```python
from build123d import *
from OCP.BRepFilletAPI import BRepFilletAPI_MakeFillet

# Parameters (mm, degrees)
SKETCH1_R                = 1.5
BOSS_EXTRUDE1_DEPTH      = 1.5
BOSS_EXTRUDE2_DEPTH      = 2
BOSS_EXTRUDE2_DEPTH_BACK = 1.5
SKETCH3_W                = 5
SKETCH3_H                = 0.7
SKETCH4_W                = 5
SKETCH4_H                = 1.5
BOSS_EXTRUDE3_DEPTH      = 0.15
FILLET2_R                = 0.85
SKETCH5_W                = 5
SKETCH5_H                = 1.2
BOSS_EXTRUDE4_DEPTH      = 2.5
BOSS_EXTRUDE4_2_DEPTH    = 2.5
SKETCH6_W                = 4
SKETCH6_H                = 5
BOSS_EXTRUDE5_DEPTH      = 2.35
FILLET3_R                = 1.5
CUT_EXTRUDE1_DEPTH       = 2.5
FILLET4_R1               = 3
FILLET4_R2               = 1


with BuildPart() as part:
    # Sketch1 → Boss-Extrude1 (new body)
    with BuildSketch(Plane(origin=(0, 0, 0), x_dir=(1, 0, 0), z_dir=(0, 1, 0))):
        with BuildLine():
            Line((0, 0), (43, 0))
            Line((43, 0), (43, 36))
            Line((43, 36), (43, 41))
            ThreePointArc((43, 41), (39, 45), (35, 41))
            Line((35, 41), (35, 36))
            Line((35, 36), (0, 36))
            Line((0, 36), (0, 0))
        make_face()
        with Locations(Location((39, 41, 0), (0, 0, 270))):
            Circle(SKETCH1_R, mode=Mode.SUBTRACT)
    extrude(amount=BOSS_EXTRUDE1_DEPTH)



with BuildPart() as body_2:
    # Sketch3 → Boss-Extrude2 (new, two sides: drawn at the far end of the back side and taken through both)
    with BuildSketch(Plane.XY.offset(-BOSS_EXTRUDE2_DEPTH_BACK)):
        with Locations((39, 2)):
            Rectangle(SKETCH3_W, SKETCH3_H)
    extrude(amount=BOSS_EXTRUDE2_DEPTH + BOSS_EXTRUDE2_DEPTH_BACK)


with BuildPart() as part_1:
    add(part.part)

    add(body_2.part)  # Boss-Extrude3 merges body 2
    # Sketch4 → Boss-Extrude3 (add)
    with BuildSketch(Plane.XZ.offset(-1.65)):
        with Locations((39, -0.75)):
            Rectangle(SKETCH4_W, SKETCH4_H)
    extrude(amount=BOSS_EXTRUDE3_DEPTH)

    # Fillet2
    fillet2_edges = [part_1.edges().sort_by_distance(p)[0] for p in [
        (39, 1.5, -1.5),
    ]]
    fillet(fillet2_edges, radius=FILLET2_R - 0.0001)  # a hair under: the kernel refuses the full size



with BuildPart() as body_2_2:
    # Sketch5 → Boss-Extrude4 (new body)
    with BuildSketch(Plane.ZY):
        with Locations((-10, 3.25)):
            Rectangle(SKETCH5_W, SKETCH5_H)
    extrude(amount=BOSS_EXTRUDE4_DEPTH)


with BuildPart() as body_3:
    # Sketch5 → Boss-Extrude4 2 (new body)
    with BuildSketch(Plane.ZY):
        with Locations((-26, 3.25)):
            Rectangle(SKETCH5_W, SKETCH5_H)
    extrude(amount=BOSS_EXTRUDE4_2_DEPTH)


with BuildPart() as part_2:
    add(part_1.part)

    add(body_2_2.part)  # Boss-Extrude5 merges body 2 2

    add(body_3.part)  # Boss-Extrude5 merges body 3
    # Sketch6 → Boss-Extrude5 (add)
    with BuildSketch(Plane(origin=(0, 1.5, 0), x_dir=(1, 0, 0), z_dir=(0, 1, 0))):
        with Locations((2, 26)):
            Rectangle(SKETCH6_W, SKETCH6_H)
        with Locations((2, 10)):
            Rectangle(SKETCH6_W, SKETCH6_H)
    extrude(amount=BOSS_EXTRUDE5_DEPTH)

    # Fillet3
    fillet3_edges = [part_2.edges().sort_by_distance(p)[0] for p in [
        (2, 1.5, -7.5),
    ]]
    fillet(fillet3_edges, radius=FILLET3_R)
    fillet3_2_edges = [part_2.edges().sort_by_distance(p)[0] for p in [
        (4, 1.5, -10),
    ]]
    fillet(fillet3_2_edges, radius=FILLET3_R)
    fillet3_3_edges = [part_2.edges().sort_by_distance(p)[0] for p in [
        (2, 1.5, -12.5),
    ]]
    fillet(fillet3_3_edges, radius=FILLET3_R)
    fillet3_4_edges = [part_2.edges().sort_by_distance(p)[0] for p in [
        (2, 1.5, -23.5),
    ]]
    fillet(fillet3_4_edges, radius=FILLET3_R)
    fillet3_5_edges = [part_2.edges().sort_by_distance(p)[0] for p in [
        (4, 1.5, -26),
    ]]
    fillet(fillet3_5_edges, radius=FILLET3_R - 0.0001)  # a hair under: the kernel refuses the full size
    fillet3_6_edges = [part_2.edges().sort_by_distance(p)[0] for p in [
        (2, 1.5, -28.5),
    ]]
    fillet(fillet3_6_edges, radius=FILLET3_R - 0.0001)  # a hair under: the kernel refuses the full size

    # Sketch7 → Cut-Extrude1 (cut)
    with BuildSketch(Plane(origin=(0, 1.5, 0), x_dir=(1, 0, 0), z_dir=(0, 1, 0))):
        Polygon((13.196152423, 29), (8, 32), (8, 26), align=None)
        Polygon((17, 26), (22.196152423, 29), (17, 32), align=None)
        Polygon((26, 26), (31.196152423, 29), (26, 32), align=None)
        Polygon((35, 26), (40.196152423, 29), (35, 32), align=None)
        Polygon((13.196152423, 18), (8, 21), (8, 15), align=None)
        Polygon((17, 15), (22.196152423, 18), (17, 21), align=None)
        Polygon((26, 15), (31.196152423, 18), (26, 21), align=None)
        Polygon((35, 15), (40.196152423, 18), (35, 21), align=None)
        Polygon((13.196152423, 7), (8, 10), (8, 4), align=None)
        Polygon((17, 4), (22.196152423, 7), (17, 10), align=None)
        Polygon((26, 4), (31.196152423, 7), (26, 10), align=None)
        Polygon((35, 4), (40.196152423, 7), (35, 10), align=None)
        Polygon((9.5, 23.5), (14.696152423, 26.5), (14.696152423, 20.5), align=None)
        Polygon((23.696152423, 20.5), (18.5, 23.5), (23.696152423, 26.5), align=None)
        Polygon((32.696152423, 20.5), (27.5, 23.5), (32.696152423, 26.5), align=None)
        Polygon((14.696152423, 9.5), (9.5, 12.5), (14.696152423, 15.5), align=None)
        Polygon((18.5, 12.5), (23.696152423, 15.5), (23.696152423, 9.5), align=None)
        Polygon((32.696152423, 9.5), (27.5, 12.5), (32.696152423, 15.5), align=None)
    extrude(amount=-CUT_EXTRUDE1_DEPTH, mode=Mode.SUBTRACT)

    # Fillet4: one fillet with a radius per group of edges: ONE call of the kernel's fillet builder (fillet() takes one radius for all edges)
    fillet4_edges_1 = [part_2.edges().sort_by_distance(p)[0] for p in [
        (0, 0.75, 0),
        (0, 0.75, -36),
    ]]
    fillet4_edges_2 = [part_2.edges().sort_by_distance(p)[0] for p in [
        (43, 0.75, 0),
    ]]
    fillet4 = BRepFilletAPI_MakeFillet(part_2.part.solid().wrapped)
    for e in fillet4_edges_1:
        fillet4.Add(FILLET4_R1, e.wrapped)
    for e in fillet4_edges_2:
        fillet4.Add(FILLET4_R2, e.wrapped)
    add(Compound.cast(fillet4.Shape()), mode=Mode.REPLACE)


solid = part_2.part
```
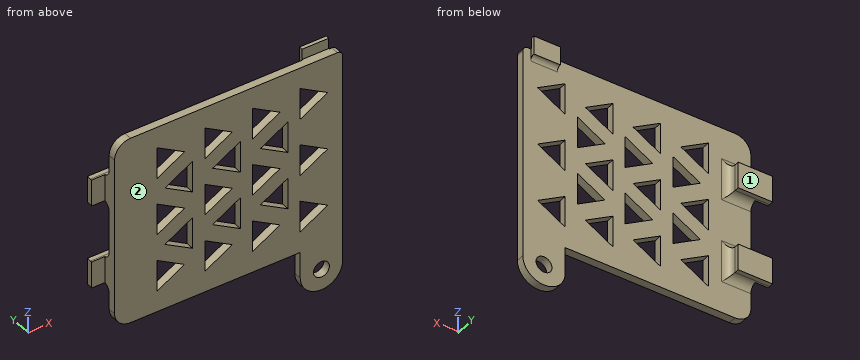
Geometry: final body of the model. Coordinates: model frame, mm. Face numbers are marked on the shaded views. Give positions to 0.01 mm unless a question says otherwise; leave off trailing zeros. Loops run counter-clockwise (first coordinate to the right, second up) from the corner with the lowest first, then second, coordinate; pieces in that order, holes last. Notation, with made-up numbers: (-29.75, 54.5) -> (5.25, 54.5) arc R16 ccw to (5.25, 71.5) -> close; hole circle Ø4 at (14, 78.5). An arc over 180 degrees is marked (long way). Use CSV: the item, a comma, the result in double quotes.
(1) Cut plane A-A (x = 39). Count the separate pieces of the cut face and the enclosed holes in it, plus the area to 3 significant figures.
From the geometry:
separate pieces,"5"
enclosed holes,"0"
area,"59.6 mm^2"
(2) Ray query, line 1 along X through (y, z) = (0.55, -41); line 2 along X through (y, z) = (1.45, -19); line 3 along Y through (x, z) = (25, -24.5). Return the intervals inside material, ascending. Write a range as [from, to].
From the geometry:
line 1,"[35, 37.5], [40.5, 43]"
line 2,"[0, 8], [11.46, 17], [20.46, 26], [29.46, 35], [38.46, 43]"
line 3,"[0, 1.5]"
(3) Cut plane B-B (x = 19.5). Output: boundary loops of the cut face in (y, z).
From the geometry:
outline,"(0, -36) -> (1.5, -36) -> (1.5, -30.56) -> (0, -30.56) -> close; (0, -27.44) -> (1.5, -27.44) -> (1.5, -24.08) -> (0, -24.08) -> close; (0, -22.92) -> (1.5, -22.92) -> (1.5, -19.56) -> (0, -19.56) -> close; (0, -16.44) -> (1.5, -16.44) -> (1.5, -13.08) -> (0, -13.08) -> close; (0, -11.92) -> (1.5, -11.92) -> (1.5, -8.56) -> (0, -8.56) -> close; (0, -5.44) -> (1.5, -5.44) -> (1.5, 0) -> (0, 0) -> close"
(4) Pull-direction query (Y, two-part tool) for the marked faces 1 and 2; classes: released by +Y, released by -Y, zero draft, split by the parting line, or undercut.
From the geometry:
face 1,"released by +Y"
face 2,"released by -Y"
(5) First-contact query: P1, Ø2, axis at x = 14, z = -37.5, coming from the +Y side; P2, Ø1.5, axis at x = 30, y = 1, coming from the -Z side; P3, Ø12, axis at x = 17, z = -35, coming from the +Y side; P4, Ø1.2, axis at y = 0.5, z = -37.5, coming from the -X side. Flat tips, straight axial feed; report the tip coordinate or a pass-through.
From the geometry:
P1,"through"
P2,"z = -36"
P3,"y = 1.5"
P4,"x = 35"
(6) Cut plane C-C (x = 29). Output: boundary loops of the cut face in (y, z).
From the geometry:
outline,"(0, -36) -> (1.5, -36) -> (1.5, -30.27) -> (0, -30.27) -> close; (0, -27.73) -> (1.5, -27.73) -> (1.5, -24.37) -> (0, -24.37) -> close; (0, -22.63) -> (1.5, -22.63) -> (1.5, -19.27) -> (0, -19.27) -> close; (0, -16.73) -> (1.5, -16.73) -> (1.5, -13.37) -> (0, -13.37) -> close; (0, -11.63) -> (1.5, -11.63) -> (1.5, -8.27) -> (0, -8.27) -> close; (0, -5.73) -> (1.5, -5.73) -> (1.5, 0) -> (0, 0) -> close"
